```python
from build123d import *

# Parameters (mm, degrees)
SKETCH1_R            = 3.125
BOSS_EXTRUDE1_DEPTH  = 2.5
BOSS_EXTRUDE2_START  = -2.5
SKETCH2_W            = 114
SKETCH2_H            = 2.5
BOSS_EXTRUDE2_DEPTH  = 6
SKETCH2_6_W          = 114
SKETCH2_6_H          = 2
BOSS_EXTRUDE3_DEPTH  = 10
SKETCH5_W            = 53
SKETCH5_H            = 15
SKETCH5_R            = 1.03775
BOSS_EXTRUDE4_DEPTH  = 2.5
CHAMFER1_SIZE        = 6.25
CHAMFER2_SIZE        = 4
FILLET2_R            = 1
FILLET3_R            = 4
CUT_EXTRUDE2_DEPTH   = 171.104117862
MOVE_START           = 2.5
MOVE_FACE1_OUTLINE_W = 114
MOVE_FACE1_OUTLINE_H = 30.7
MOVE_FACE1_OUTLINE_R = 3.125
MOVE_FACE1_DEPTH     = 0.5
MOVE_FACE2_BY        = 1
MOVE_FACE3_BY        = 0.5
MOVE_FACE4_BY        = 0.65


# Read off the part's stored shape, not the designer's step: Move Face1
with BuildPart() as part:
    # Sketch1 → Boss-Extrude1 (new body)
    with BuildSketch(Plane.XY):
        Polygon((52.096119502, 0), (52.096119502, 25.2), (52.096119502, 28.2), (166.096119502, 28.2), (166.096119502, 25.2), (166.096119502, 0), (166.096119502, -2.5), (52.096119502, -2.5), align=None)
        with Locations((84.096119502, 12.6)):
            Circle(SKETCH1_R, mode=Mode.SUBTRACT)
        with Locations((134.096119502, 12.6)):
            Circle(SKETCH1_R, mode=Mode.SUBTRACT)
        with Locations((59.096119502, 12.6)):
            Circle(SKETCH1_R, mode=Mode.SUBTRACT)
        with Locations((159.096119502, 12.6)):
            Circle(SKETCH1_R, mode=Mode.SUBTRACT)
    extrude(amount=BOSS_EXTRUDE1_DEPTH)

    # Sketch2 → Boss-Extrude2 (add)
    with BuildSketch(Plane.XY.offset(2.5).offset(BOSS_EXTRUDE2_START)):
        with Locations((109.096119502, -1.25)):
            Rectangle(SKETCH2_W, SKETCH2_H)
    extrude(amount=-BOSS_EXTRUDE2_DEPTH)

    # Sketch2<6> → Boss-Extrude3 (add)
    with BuildSketch(Plane.XY.offset(2.5)):
        with Locations((109.096119502, 27.2)):
            Rectangle(SKETCH2_6_W, SKETCH2_6_H)
    extrude(amount=-BOSS_EXTRUDE3_DEPTH)

    # Sketch5 → Boss-Extrude4 (add)
    with BuildSketch(Plane.XZ.offset(2.5)):
        with Locations((139.596119502, -13.5)):
            Rectangle(SKETCH5_W, SKETCH5_H)
        with Locations((146.088533212, -17.095733919)):
            Circle(SKETCH5_R, mode=Mode.SUBTRACT)
        with Locations((132.088533212, -17.095733919)):
            Circle(SKETCH5_R, mode=Mode.SUBTRACT)
    boss_extrude4 = extrude(amount=-BOSS_EXTRUDE4_DEPTH)

    # Mirror1: Boss-Extrude4 across plane
    add(boss_extrude4.mirror(Plane(origin=(109.096119502, 0, 0), x_dir=(0, 0, 1), z_dir=(1, 0, 0))))

    # Chamfer1
    chamfer1_edges = [part.edges().sort_by_distance(p)[0] for p in [
        (166.096119502, -1.25, -21),
        (113.096119502, -1.25, -21),
        (52.096119502, -1.25, -21),
        (105.096119502, -1.25, -21),
    ]]
    chamfer(chamfer1_edges, length=CHAMFER1_SIZE)

    # Chamfer2
    chamfer2_edges = [part.edges().sort_by_distance(p)[0] for p in [
        (52.096119502, 27.2, -7.5),
        (166.096119502, 27.2, -7.5),
    ]]
    chamfer(chamfer2_edges, length=CHAMFER2_SIZE)

    # Fillet2
    fillet2_edges = [part.edges().sort_by_distance(p)[0] for p in [
        (98.846119502, -1.25, -21),
        (105.096119502, -1.25, -14.75),
        (113.096119502, -1.25, -14.75),
        (159.846119502, -1.25, -21),
        (119.346119502, -1.25, -21),
        (166.096119502, -1.25, -14.75),
        (166.096119502, 27.2, -3.5),
        (56.096119502, 27.2, -7.5),
        (162.096119502, 27.2, -7.5),
        (52.096119502, 27.2, -3.5),
        (52.096119502, -1.25, -14.75),
    ]]
    fillet(fillet2_edges, radius=FILLET2_R)

    # Fillet3
    fillet3_edges = [part.edges().sort_by_distance(p)[0] for p in [
        (113.096119502, -1.25, -6),
        (105.096119502, -1.25, -6),
    ]]
    fillet(fillet3_edges, radius=FILLET3_R - 0.0001)  # a hair under: the kernel refuses the full size

    # Sketch6 → Cut-Extrude2 (cut, through all)
    with BuildSketch(Plane.XY.offset(2.5)):
        with BuildLine():
            Line((119.096119502, 24.5), (99.096119502, 24.5))
            ThreePointArc((99.096119502, 24.5), (96.096119502, 21.5), (99.096119502, 18.5))
            Line((99.096119502, 18.5), (119.096119502, 18.5))
            ThreePointArc((119.096119502, 18.5), (122.096119502, 21.5), (119.096119502, 24.5))
        make_face()
    extrude(amount=-CUT_EXTRUDE2_DEPTH, mode=Mode.SUBTRACT)

    # Move Face1 outline → Move Face1 (add)
    with BuildSketch(Plane.XY.offset(MOVE_START)):
        with Locations((109.096119502, 12.85)):
            Rectangle(MOVE_FACE1_OUTLINE_W, MOVE_FACE1_OUTLINE_H)
        with Locations((59.096119502, 12.6)):
            Circle(MOVE_FACE1_OUTLINE_R, mode=Mode.SUBTRACT)
        with Locations((84.096119502, 12.6)):
            Circle(MOVE_FACE1_OUTLINE_R, mode=Mode.SUBTRACT)
        with Locations((134.096119502, 12.6)):
            Circle(MOVE_FACE1_OUTLINE_R, mode=Mode.SUBTRACT)
        with Locations((159.096119502, 12.6)):
            Circle(MOVE_FACE1_OUTLINE_R, mode=Mode.SUBTRACT)
        with BuildLine():
            Line((99.096119502, 24.5), (119.096119502, 24.5))
            ThreePointArc((119.096119502, 24.5), (122.096119502, 21.5), (119.096119502, 18.5))
            Line((119.096119502, 18.5), (99.096119502, 18.5))
            ThreePointArc((99.096119502, 18.5), (96.096119502, 21.5), (99.096119502, 24.5))
        make_face(mode=Mode.SUBTRACT)
    extrude(amount=MOVE_FACE1_DEPTH)

    # Move Face2: a face moved outward by 1.0
    extrude(part.faces().sort_by_distance((109.096119502, 26.2, -3.703733506))[0], amount=MOVE_FACE2_BY, dir=(0, -1, 0))

    # Move Face3: a face moved inward by 0.5
    extrude(part.faces().sort_by_distance((109.096119502, 28.2, -2.196700016))[0], amount=MOVE_FACE3_BY, dir=(0, -1, 0), mode=Mode.SUBTRACT)

    # Move Face4: a face moved inward by 0.65
    extrude(part.faces().sort_by_distance((109.096119502, -2.5, -3))[0], amount=MOVE_FACE4_BY, dir=(0, 1, 0), mode=Mode.SUBTRACT)


solid = part.part
```
Work out the finished part from the listing and answer in its coordinate system (mm). A direction names the side the tool comes from. Round coordinates to 2 decimals unless told otherwise and drop trailing zeros. Write each loop counter-clockwise with the first axis right and the second up, starting at its lowest first coordinate (ties: lowest second). Pieces come first, ordered by that corner, then holes. Notation, with made-up numbers: (5, 34) -> (23, 34) arc R14 ccw to (23, 55) -> close; hole circle Ø5 at (-33, -9). An arc over 180 degrees is marked (long way). Write each question's results on one line, items separated by ' | '.
Q1. Section B-B, the plane z = -11 is taken. Write down the section's boundary in (x, y).
Data:
outline: (52.1, -1.85) -> (105.1, -1.85) -> (105.1, 0) -> (52.1, 0) -> close; (113.1, -1.85) -> (166.1, -1.85) -> (166.1, 0) -> (113.1, 0) -> close
Q2. Flat-ended cylindrical pins translate along their axes: P1, Ø4, axis at x = 159.1, y = 12.6, coming from the +Z side (1 decimal); P2, Ø10, axis at x = 134.1, y = 12.6, coming from the -Z side; P3, Ø2.5, axis at x = 72.1, z = -17.1, coming from the +Y side. Find the tip coordinate at first contact, or state that the pin passes through.
Data:
P1: through | P2: z = 0 | P3: y = 0
Q3. Section A-A, the plane y = 21.5 is taken. Write down the section's boundary in (x, z), then the cut area to 3 significant figures.
Data:
outline: (52.1, 0) -> (96.1, 0) -> (96.1, 3) -> (52.1, 3) -> close; (122.1, 0) -> (166.1, 0) -> (166.1, 3) -> (122.1, 3) -> close | area: 264 mm^2
Q4. Section C-C, the plane x = 61 is taken. Write down the section's boundary in (y, z).
Data:
outline: (-1.85, -21) -> (0, -21) -> (0, 0) -> (10.12, 0) -> (10.12, 3) -> (-1.85, 3) -> close; (15.08, 0) -> (25.2, 0) -> (25.2, -7.5) -> (27.7, -7.5) -> (27.7, 3) -> (15.08, 3) -> close
Q5. Straight lines are drawn through the part: line 1 along Y through (x, z) = (59, -5.5); line 2 along Z through (x, y) = (117, 7); line 3 along Y through (x, z) = (107, -7.25). For each, find the intervals that lie inside material, in ascending order. Write a range as [from, to].
Data:
line 1: [-1.85, 0], [25.2, 27.7] | line 2: [0, 3] | line 3: [25.2, 27.7]
Q6. Which of the six approach directions +Z, -Z, +X, -X, +Y, -Y give full straight-line access (tool end or side, diameter ignored) to faces 1 (the flat face through (110, 13, 0)), 2 (the flat face through (54.072, 26.468, -5.476)), 3 (the flat face through (113.096, -1, -12))?
Data:
face 1: -Z, +X, -X | face 2: -Z, -X, +Y | face 3: -Z, +Y, -Y
Q7. Section D-D, the plane y = 12.6 is taken. Write down the section's boundary in (x, z).
Data:
outline: (52.1, 0) -> (55.97, 0) -> (55.97, 3) -> (52.1, 3) -> close; (62.22, 0) -> (80.97, 0) -> (80.97, 3) -> (62.22, 3) -> close; (87.22, 0) -> (130.97, 0) -> (130.97, 3) -> (87.22, 3) -> close; (137.22, 0) -> (155.97, 0) -> (155.97, 3) -> (137.22, 3) -> close; (162.22, 0) -> (166.1, 0) -> (166.1, 3) -> (162.22, 3) -> close
Q8. Determine the mould class of faces 4 (the cylindrical face through (96.097, 21.434, 1.479)), 5 (the flat face through (108, 26, -7.5)), 6 (the flat face through (108, -1.85, -4)) for opening direction Y: released by +Y, released by -Y, zero draft, split by the parting line, or undercut.
Data:
face 4: undercut | face 5: zero draft | face 6: released by -Y
